Study the drawing (mm; zero at the part's minimum x, y, z) and answer. A direction names the side the tool comes from. Round coordinates to 2 decimals unless told otherwise and drop trailing zeros. Order: outer loops, then holes, each group sorted by start corner. A loop starts at its lowest first (then second) coordinate and runs counter-clockwise, first axis right, second up. Notation, with made-up numbers: M 80.25,68.5 L 92.25,68.5 A24 ccw 92.25,93.5 Z; hole C 17.5,78 d9. An arc over 180 degrees is marked long. Put each result on its own line as item: value. Start each with the question number.
1. The part is cut by section D-D (y = 1.5). Give the vertices of the cut face in (x, z) (1 decimal), then the cut area to 3 significant figures.
2. The part is cut by section B-B (x = 6.35). Give the vertices of the cut face in (y, z).
3. The mould has two halves that part along X. Classify the marked faces 1, 2 and 3: +X half, -X half, draft (parallel to the pull), parting line (faces both ways), or undercut.
4. Consider line 1 (Y direction, x = 6.35, z = 3); line 2 (X direction, y = 3.75, z = 6) (1 decimal); line 3 (X direction, y = 6, z = 2.75) (1 decimal). Determine where each line is inside the solid, lowest interval first.
5. Which of the six approach directions +Z, -Z, +X, -X, +Y, -Y give full straight-line access (tool end or side, diameter ignored) to the marked faces 4, 5 and 6?
6. Each of these flat-tipped pins is pushed along its axis until it touches: pin 1 Ø6 at (y, z) = (1.5, 10.5) entering from -X; pin 2 Ø4.5 at (x, y) = (6.35, 6.35) entering from +Z; pin 3 Ø6.5 at (x, z) = (23.5, 6.5) entering from -Y. Where does it stop, or does it pass through?
7. The part is cut by section C-C (y = 6.35). Give the vertices of the cut face in (x, z) (1 decimal).
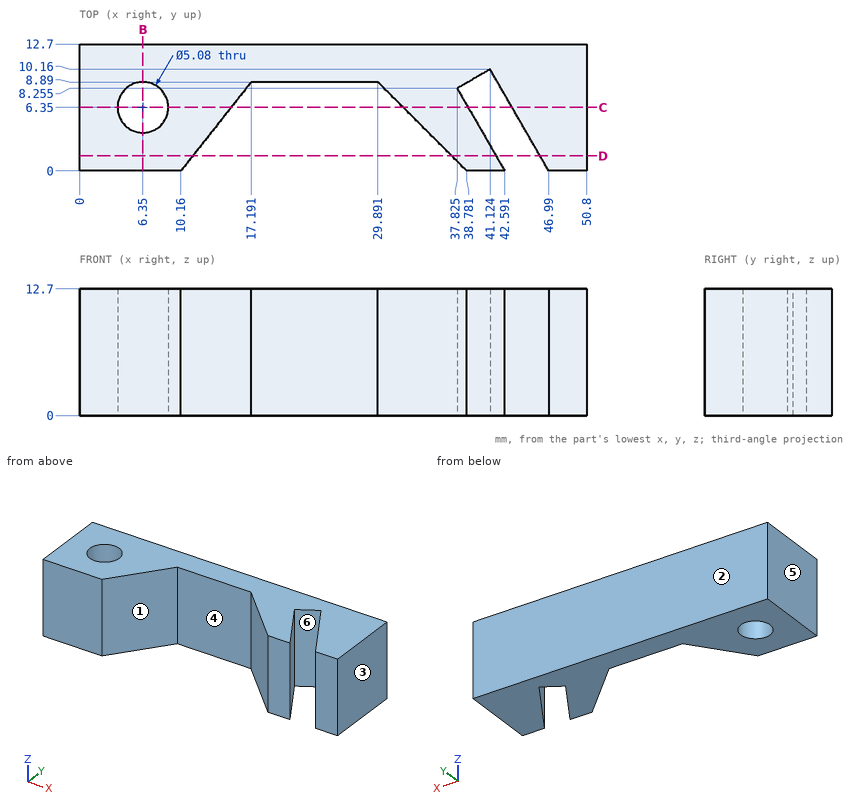
Resolved:
1. outline: M 0,0 L 11.3,0 L 11.3,12.7 L 0,12.7 Z; M 37.3,0 L 41.7,0 L 41.7,12.7 L 37.3,12.7 Z; M 46.1,0 L 50.8,0 L 50.8,12.7 L 46.1,12.7 Z
1. area: 260 mm2
2. outline: M 0,0 L 3.81,0 L 3.81,12.7 L 0,12.7 Z; M 8.89,0 L 12.7,0 L 12.7,12.7 L 8.89,12.7 Z
3. face 1: undercut
3. face 2: draft
3. face 3: +X half
4. line 1: 0 to 3.81, 8.89 to 12.7
4. line 2: 0 to 13.1, 35 to 40.4, 44.8 to 50.8
4. line 3: 0 to 3.8, 8.9 to 14.9, 32.8 to 39.1, 43.5 to 50.8
5. face 4: +Z, -Z, -Y
5. face 5: +Z, -Z, -X, +Y, -Y
5. face 6: +Z, -Z
6. pin 1: x = 0
6. pin 2: through
6. pin 3: y = 8.89
7. outline: M 0,0 L 3.8,0 L 3.8,12.7 L 0,12.7 Z; M 8.9,0 L 15.2,0 L 15.2,12.7 L 8.9,12.7 Z; M 32.4,0 L 38.9,0 L 38.9,12.7 L 32.4,12.7 Z; M 43.3,0 L 50.8,0 L 50.8,12.7 L 43.3,12.7 Z
